Design review of the part built by this model. Coordinates are the model's own, in mm. A direction names the side the tool comes from. Give positions to 0.01 mm unless a question says otherwise; leave off trailing zeros. Loops run counter-clockwise (first coordinate to the right, second up) from the corner with the lowest first, then second, coordinate; pieces in that order, holes last. Notation, with made-up numbers: (-30.75, 20.5) -> (-20.75, 20.5) arc R9 ccw to (-20.75, 37.5) -> close; hole circle Ø1 at (7.5, 42). An arc over 180 degrees is marked (long way). Use a Markdown table: item, result. Add a question column.
1. To check wall thickness, follow line 1 (Y direction, x = 27.5, z = -10); line 2 (Y direction, x = -25.5, z = -2); line 3 (Z direction, x = 4, y = 44). State the ranges of each line that lie inside material, in increasing order.
2. Add section B-B (z = 0). State the section outline as (x, y) points.
3. Add section C-C (y = 37). State the section outline as (x, z) points.
4. Add section D-D (y = 9). State the section outline as (x, z) points.
5. Add section A-A (x = 0). State the section outline as (y, z) points, and give its area (3 significant figures).
6. For faces 1 (the flat face through (12, -30, 0)), 2 (the cylindrical face through (26.327, 27.465, -10.916)), 3 (the flat face through (0, -50, 0)), list the 3-axis set-ups (+Z, -Z, +X, -X, +Y, -Y) from which the entire face can be reached by the end or side of a thin tool; tool diameter is ignored.
7. For pin 1 Ø2 at (x, y) = (-34, 7) entering from +Z; pin 2 Ø1 at (x, z) = (51, 2) entering from -Y; pin 3 Ø5 at (x, y) = (18, 10.5) entering from +Z, all flat-tipped, find the tip position at first contact; note any pin that passes through.
```python
from build123d import *

# Parameters (mm, degrees)
F0_R     = 80
F0_R_2   = 75
F0_R_3   = 28.5
F1_DEPTH = 25
F0_R_4   = 10
F2_DEPTH = 30
F3_DEPTH = 50
F4_R     = 5
F5_SIZE  = 1


with BuildPart() as f1:
    # F0 (on Front) → F1 (new body, symmetric)
    with BuildSketch(Plane.XZ):
        Circle(F0_R)
        Circle(F0_R_2, mode=Mode.SUBTRACT)
        Circle(F0_R_2)
        Circle(F0_R_3, mode=Mode.SUBTRACT)
    extrude(amount=F1_DEPTH, both=True)

    # F0 (on Front) → F2 (join, symmetric)
    with BuildSketch(Plane.XZ):
        Circle(F0_R_3)
        Circle(F0_R_4, mode=Mode.SUBTRACT)
    extrude(amount=F2_DEPTH, both=True)

    # F0 (on Front) → F3 (join, symmetric)
    with BuildSketch(Plane.XZ):
        Circle(F0_R_4)
    extrude(amount=F3_DEPTH, both=True)

    # F4
    f4_edges = [f1.edges().sort_by_distance(p)[0] for p in [
        (-80, -25, 0),
        (-80, 25, 0),
    ]]
    fillet(f4_edges, radius=F4_R)

    # F5
    f5_edges = [f1.edges().sort_by_distance(p)[0] for p in [
        (-10, -50, 0),
        (-10, 50, 0),
    ]]
    chamfer(f5_edges, length=F5_SIZE)


solid = f1.part
```
Taken from the geometry:
| question | item | result |
|---|---|---|
| 1 | line 1 | y = -25 to 25 |
| 1 | line 2 | y = -30 to 30 |
| 1 | line 3 | z = -9.17 to 9.17 |
| 2 | outline | (-80, -20) arc R5 ccw to (-75, -25) -> (-28.5, -25) -> (-28.5, -30) -> (-10, -30) -> (-10, -49) -> (-9, -50) -> (9, -50) -> (10, -49) -> (10, -30) -> (28.5, -30) -> (28.5, -25) -> (75, -25) arc R5 ccw to (80, -20) -> (80, 20) arc R5 ccw to (75, 25) -> (28.5, 25) -> (28.5, 30) -> (10, 30) -> (10, 49) -> (9, 50) -> (-9, 50) -> (-10, 49) -> (-10, 30) -> (-28.5, 30) -> (-28.5, 25) -> (-75, 25) arc R5 ccw to (-80, 20) -> close |
| 3 | outline | circle Ø20 at (0, 0) |
| 4 | outline | circle Ø160 at (0, 0) |
| 5 | outline | (-50, -9) -> (-49, -10) -> (-30, -10) -> (-30, -28.5) -> (-25, -28.5) -> (-25, -75) arc R5 ccw to (-20, -80) -> (20, -80) arc R5 ccw to (25, -75) -> (25, -28.5) -> (30, -28.5) -> (30, -10) -> (49, -10) -> (50, -9) -> (50, 9) -> (49, 10) -> (30, 10) -> (30, 28.5) -> (25, 28.5) -> (25, 75) arc R5 ccw to (20, 80) -> (-20, 80) arc R5 ccw to (-25, 75) -> (-25, 28.5) -> (-30, 28.5) -> (-30, 10) -> (-49, 10) -> (-50, 9) -> close |
| 5 | area | 9,350 mm^2 |
| 6 | face 1 | -Y |
| 6 | face 2 | +Y |
| 6 | face 3 | +Z, -Z, +X, -X, -Y |
| 7 | pin 1 | stops at z = 72.88 |
| 7 | pin 2 | stops at y = -25 |
| 7 | pin 3 | stops at z = 78.48 |
